The figure shows three views and two pictorial views of one solid part (mm, origin at its lowest corner). Answer the questions. A direction names the side the tool comes from. Coordinates: 2 decimals unless noted, no trailing zeros. Order: outer loops, then holes, each group sorted by start corner. A loop starts at its lowest first (then second) coordinate and runs counter-clockwise, first axis right, second up.
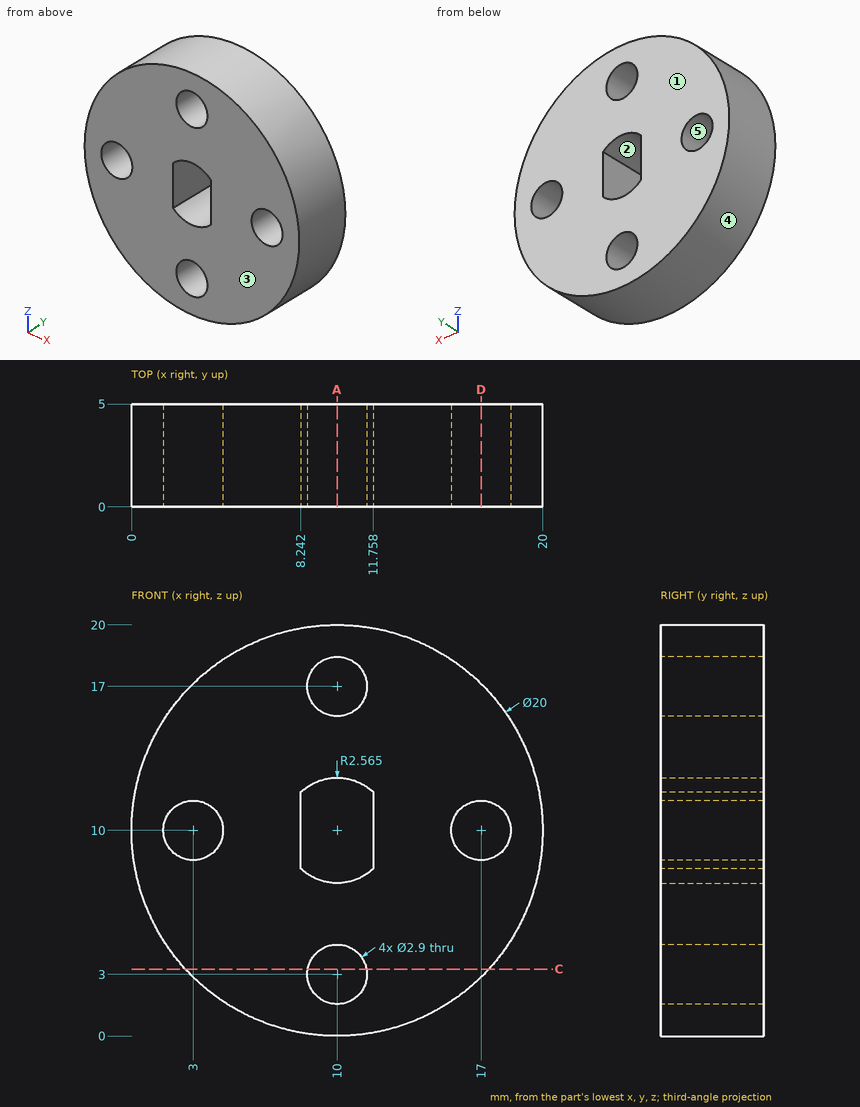
Q1. The part is cut by section A-A, the plane x = 10. State how many separate pieces and enclosed holes the cut face has.
Q2. The part is cut by section D-D, the plane x = 17. Determine the outline of the cut face in (y, z).
Q3. Which of the six approach directions +Z, -Z, +X, -X, +Y, -Y give full straight-line access (tool end or side, diameter ignored) to the marked faces 1 and 2?
Q4. Each of these flat-tipped pins is pushed along its axis until it touches: P1, Ø1, axis at y = 1.5, z = 3.5, coming from the -X side; P2, Ø1.5, axis at x = 14.5, y = 0.5, coming from the -Z side; P3, Ø1.5, axis at x = 13.5, y = 0.5, coming from the -Z side (1 decimal); P4, Ø2.5, axis at x = 10, z = 17, coming from the -Y side. Where does it stop, or does it pass through?
Q5. The part is cut by section C-C, the plane z = 3.25. Determine the outline of the cut face in (x, y).
Q6. Straight lines are drawn through the part: L1, parallel to X at y = 3, z = 10; L2, parallel to X at y = 2.95, z = 17; L3, parallel to X at y = 3.15, z = 17.25 (1 decimal). For each, find the intervals that lie inside material, in ascending order.
Q7. Determine the mould class of the marked faces 3, 4 and 5 for opening direction Z: +Z half, -Z half, draft (parallel to the pull), parting line (faces both ways), or undercut.
Computed values:
1. separate pieces: 4
1. enclosed holes: 0
2. outline: (0, 2.86) - (5, 2.86) - (5, 8.55) - (0, 8.55) - close; (0, 11.45) - (5, 11.45) - (5, 17.14) - (0, 17.14) - close
3. face 1: +Z, -Z, +X, -X, +Y
3. face 2: +Y, -Y
4. P1: stops at x = 2
4. P2: stops at z = 0.73
4. P3: stops at z = 0.4
4. P4: passes through
5. outline: (2.62, 0) - (8.57, 0) - (8.57, 5) - (2.62, 5) - close; (11.43, 0) - (17.38, 0) - (17.38, 5) - (11.43, 5) - close
6. L1: x = 0 to 1.55, 4.45 to 8.24, 11.76 to 15.55, 18.45 to 20
6. L2: x = 2.86 to 8.55, 11.45 to 17.14
6. L3: x = 3.1 to 8.6, 11.4 to 16.9
7. face 3: draft
7. face 4: parting line
7. face 5: undercut
